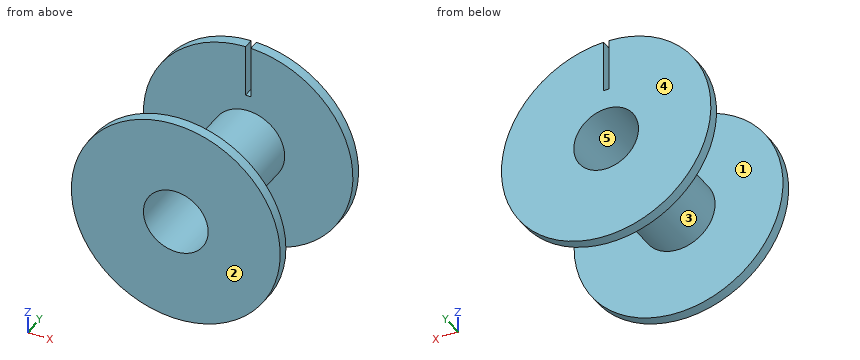
from build123d import *

# Parameters (mm, degrees)
EXTRUDE_3_DEPTH     = 2
SKETCH_5_R          = 6.2
CUT_EXTRUDE_2_DEPTH = 2
SKETCH_6_R          = 7
EXTRUDE_6_DEPTH     = 23.5
SKETCH_7_R          = 6.2
CUT_EXTRUDE_3_DEPTH = 23.5
SKETCH_8_R          = 20
EXTRUDE_7_DEPTH     = 2
SKETCH_9_R          = 6.2
CUT_EXTRUDE_4_DEPTH = 2


with BuildPart() as part:
    # 草图3 → 凸台-拉伸3 (new body)
    with BuildSketch(Plane(origin=(0, 0, 0), x_dir=(1, 0, 0), z_dir=(0, 1, 0))):
        with BuildLine():
            Line((-0.5, -20.052167872), (-0.5, -10.058400643))
            Line((-0.5, -10.058400643), (0.5, -10.058400643))
            Line((0.5, -10.058400643), (0.5, -20.052167872))
            ThreePointArc((0.5, -20.052167872), (0, 20.058400643), (-0.5, -20.052167872))
        make_face()
    extrude(amount=EXTRUDE_3_DEPTH)

    # 草图5 → 切除-拉伸2 (cut)
    with BuildSketch(Plane(origin=(0, 2, 0), x_dir=(1, 0, 0), z_dir=(0, 1, 0))):
        Circle(SKETCH_5_R)
    extrude(amount=-CUT_EXTRUDE_2_DEPTH, mode=Mode.SUBTRACT)

    # 草图6 → 凸台-拉伸6 (add)
    with BuildSketch(Plane(origin=(0, 0, 0), x_dir=(-1, 0, 0), z_dir=(0, -1, 0))):
        Circle(SKETCH_6_R)
    extrude(amount=EXTRUDE_6_DEPTH)

    # 草图7 → 切除-拉伸3 (cut)
    with BuildSketch(Plane(origin=(0, 0, 0), x_dir=(1, 0, 0), z_dir=(0, 1, 0))):
        Circle(SKETCH_7_R)
    extrude(amount=-CUT_EXTRUDE_3_DEPTH, mode=Mode.SUBTRACT)

    # 草图8 → 凸台-拉伸7 (add)
    with BuildSketch(Plane.XZ.offset(23.5)):
        Circle(SKETCH_8_R)
    extrude(amount=EXTRUDE_7_DEPTH)

    # 草图9 → 切除-拉伸4 (cut)
    with BuildSketch(Plane.XZ.offset(25.5)):
        Circle(SKETCH_9_R)
    extrude(amount=-CUT_EXTRUDE_4_DEPTH, mode=Mode.SUBTRACT)


solid = part.part
Could you check a few things on this model? Use its own coordinates, in mm. Face numbers are marked on the shaded views. A direction names the side the tool comes from. Give positions to 0.01 mm unless a question says otherwise; leave off trailing zeros. Order: outer loops, then holes, each group sorted by start corner. A loop starts at its lowest first (then second) coordinate and runs counter-clockwise, first axis right, second up.
Item 1: I need wall thicknesses on line 1 (Y direction, x = -7.5, z = 5.5); line 2 (X direction, y = -9.5, z = 0); line 3 (X direction, y = -7.25, z = -5). Which ranges of each line are inside material? Lowest first, please.
Item 2: If we section it at A-A, the plane z = 0: Write out the boundary of the cut face in (x, y).
Item 3: If we mould it in two halves opening along X, with no side actions, what happens to the marked faces 3, 4 and 5? For each: pulls with the +X half, pulls with the -X half, needs draft (parallel to the pull), parting line crosses it, or undercut.
Item 4: If we section it at D-D, the plane z = 16.5: Write out the boundary of the cut face in (x, y), plus the area to 3 significant figures.
Item 5: I'm going to push flat-ended pins straight in: pin 1 (10 mm diameter, centred on x = -5.5, y = -13.5, fed in from -Z); pin 2 (1 mm diameter, centred on y = 1, z = 13, fed in from +X); pin 3 (4 mm diameter, centred on y = -15, z = -3, fed in from -X). Where does each tip first touch, or does it pass through?
Item 6: For the marked faces 1 and 2, which set-ups out of +Z, -Z, +X, -X, +Y, -Y let a thin tool reach every point of the face, with its end or its side?
Item 7: If we section it at B-B, the plane x = -1.5: Write out the boundary of the cut face in (y, z), plus the area to 3 significant figures.
Item 8: If we section it at C-C, the plane y = -15.25: Write out the boundary of the cut face in (x, z).
Values:
1. line 1: y = -25.5 to -23.5, 0 to 2
1. line 2: x = -7 to -6.2, 6.2 to 7
1. line 3: x = -4.9 to -3.67, 3.67 to 4.9
2. outline: (-20.06, 0) - (-7, 0) - (-7, -23.5) - (-20, -23.5) - (-20, -25.5) - (-6.2, -25.5) - (-6.2, 2) - (-20.06, 2) - close; (6.2, -25.5) - (20, -25.5) - (20, -23.5) - (7, -23.5) - (7, 0) - (20.06, 0) - (20.06, 2) - (6.2, 2) - close
3. face 3: parting line crosses it
3. face 4: needs draft
3. face 5: undercut
4. outline: (-11.41, 0) - (-0.5, 0) - (-0.5, 2) - (-11.41, 2) - close; (-11.3, -25.5) - (11.3, -25.5) - (11.3, -23.5) - (-11.3, -23.5) - close; (0.5, 0) - (11.41, 0) - (11.41, 2) - (0.5, 2) - close
4. area: 88.8 mm2
5. pin 1: stops at z = -6.98
5. pin 2: stops at x = 15.69
5. pin 3: stops at x = -6.93
6. face 1: none
6. face 2: +Z, -Z, +X, -X, -Y
7. outline: (-25.5, -19.94) - (-23.5, -19.94) - (-23.5, -6.84) - (0, -6.84) - (0, -20) - (2, -20) - (2, -6.02) - (-25.5, -6.02) - close; (-25.5, 6.02) - (2, 6.02) - (2, 20) - (0, 20) - (0, 6.84) - (-23.5, 6.84) - (-23.5, 19.94) - (-25.5, 19.94) - close
7. area: 150 mm2
8. outline: circle Ø14 at (0, 0); hole circle Ø12.4 at (0, 0)
